Autodesk Inventor part; units mm, degrees
ref_plane "YZ Plane" through (0, 0, 0) normal (1, 0, 0) x (0, 1, 0)
ref_plane "XZ Plane" through (0, 0, 0) normal (0, 1, 0) x (-1, 0, 0)
ref_plane "XY Plane" through (0, 0, 0) normal (0, 0, 1) x (1, 0, 0)
sketch "Sketch1" plane through (0, 0, 0) normal (1, 0, 0) x (0, 1, 0)
  circle A0 centre (0, 0) radius 1.0033
  line L0 (-1.249071, 1.652114) -> (1.249071, 1.652114)
  line L1 (1.249071, 1.652114) -> (1.249071, -1.652114)
  line L2 (1.249071, -1.652114) -> (-1.249071, -1.652114)
  line L3 (-1.249071, -1.652114) -> (-1.249071, 1.652114)
  line L4 (-1.249071, 1.652114) -> (1.249071, -1.652114) construction
  line L5 (1.249071, 1.652114) -> (-1.249071, -1.652114) construction
  dimension "d0" = 2.0066
  dimension "d1" = 37.0909
  dimension "d2" = 2.49814
extrude "Extrusion1" add sketch "Sketch1" along normal blind 3
sketch "Sketch2" plane through (0, -1.249071, -1.652114) normal (0, 0, -1) x (-1, 0, 0)
  line L0 (0, 0) -> (0, 2.498142)
  line L1 (-3.026642, 0) -> (0, 0)
  line L2 (0, 0) -> (0, 2.498142)
  line L3 (0, 2.498142) -> (-3.026642, 2.498142)
  line L4 (-3.026642, 2.498142) -> (-3.026642, 0)
  line L5 (-3.026642, 0) -> (0, 2.498142) construction
  line L6 (0, 0) -> (-3.026642, 2.498142) construction
  point P0 (0, 1.249071)
  point P1 (-1.513321, 1.249071)
  dimension "d5" = 50.4643
  dimension "d6" = 3.02664
extrude "Extrusion2" add sketch "Sketch2" along normal blind 30
draft "FaceDraft1" angle 1 pull direction (0, 0, -1) faces at (1, -1.249071, -10.550705) (3.026642, 0.416357, -21.652114) (1, 1.249071, -10.550705) fixed edges at (1.513321, -1.249071, -31.652114) (3.026642, 0, -31.652114) (1.513321, 1.249071, -31.652114)
sketch "Sketch3" plane through (0, -1.249071, -31.652114) normal (0, 0, -1) x (-1, 0, 0)
  line L0 (0, 2.491731) -> (-3, -0.000251)
  line L1 (-3, 3.079469) -> (-3, -0.581327)
  line L2 (-3.026642, 0) -> (0, 0)
  line L3 (-3, 2.491731) -> (0, 0)
  circle A0 centre (-1.5, 1.245866) radius 0.5
  point P0 (0, 1.249071)
  dimension "d10" = 1
extrude "Extrusion3" add sketch "Sketch3" along normal blind 5 contours A0 L3 L0 | L0 L3 A0 | L3 A0 L0 | L0 A0 L3
properties part number "bout tournant"
Work out the finished part from the listing and answer in its coordinate system (mm). A direction names the side the tool comes from. Coordinates: 2 decimals unless noted, no trailing zeros. Write each loop counter-clockwise with the first axis right and the second up, starting at its lowest first coordinate (ties: lowest second). Pieces come first, ordered by that corner, then holes. Notation, with made-up numbers: M -2,-19 L 25,-19 A25 ccw 25,13 Z; hole C 51,50.5 d6. An arc over 180 degrees is marked long. Answer as CSV lines item,"result". Start each with the question number.
Item 1: Consider L1, parallel to Z at x = 1.7, y = 0; L2, parallel to Z at x = 0.7, y = 0; L3, parallel to X at y = -0.7, z = -31.5. Determine where each line is inside the solid, lowest interval first.
Item 2: A tool of negligible diameter and unlimited length cuts with its end or side. For faces 4 (the face through (1, 0, 1.652)), 5 (the face through (2, 0, -34)), from which of +Z, -Z, +X, -X, +Y, -Y can it reach the whole face along a straight path? Write none if from no direction.
Item 3: Flat-ended cylindrical pins translate along their axes: P1, Ø0.6, axis at x = 3.5, y = 0, coming from the +Z side; P2, Ø1, axis at y = -1, z = -7.5, coming from the +X side; P3, Ø2, axis at y = -0.5, z = -29.5, coming from the +X side; P4, Ø1.8, axis at y = 0, z = 0, coming from the +X side. Find the tip coordinate at first contact, or state that the pin passes through.
Item 4: Determine the mould class of faces 1 (the face through (1.48, -0.74, -0.68)), 2 (the face through (1.5, 0, -36.652)), 3 (the face through (3, -1, 1)) for opening direction Z: released by +Z, released by -Z, zero draft, split by the parting line, or undercut.
Item 5: Section A-A on x = 1.5 is taken. Write down the section's boundary in (y, z).
Item 6: Section C-C on z = -4 is taken. Write down the section's boundary in (x, y), and give its area (3 significant figures).
Item 7: Section D-D on z = -24 is taken. Write down the section's boundary in (x, y), and give its area (3 significant figures).
Item 8: Section B-B on z = 0 is taken. Write down the section's boundary in (x, y), and give its area (3 significant figures).
Checks:
1,L1,"z = -36.65 to -1, 1 to 1.65"
1,L2,"z = -31.65 to -1, 1 to 1.65"
1,L3,"x = 0 to 3.03"
2,face 4,"+Z, +X, -X, +Y, -Y"
2,face 5,"-Z"
3,P1,"stops at z = -1.65"
3,P2,"stops at x = 3.46"
3,P3,"stops at x = 3.08"
3,P4,"passes through"
4,face 1,"undercut"
4,face 2,"released by -Z"
4,face 3,"zero draft"
5,outline,"M -1.83,1.65 L -1.25,-31.65 L -0.5,-31.65 L -0.5,-36.65 L 0.5,-36.65 L 0.5,-31.65 L 1.25,-31.65 L 1.83,1.65 Z; hole C 0,0 d2.01"
6,outline,"M 0,-1.73 L 3.51,-1.73 L 3.51,1.73 L 0,1.73 Z"
6,area,"12.2 mm²"
7,outline,"M 0,-1.38 L 3.16,-1.38 L 3.16,1.38 L 0,1.38 Z"
7,area,"8.74 mm²"
8,outline,"M 0,-1.8 L 3,-1.8 L 3,-1 L 0,-1 Z; M 0,1 L 3,1 L 3,1.8 L 0,1.8 Z"
8,area,"4.79 mm²"
